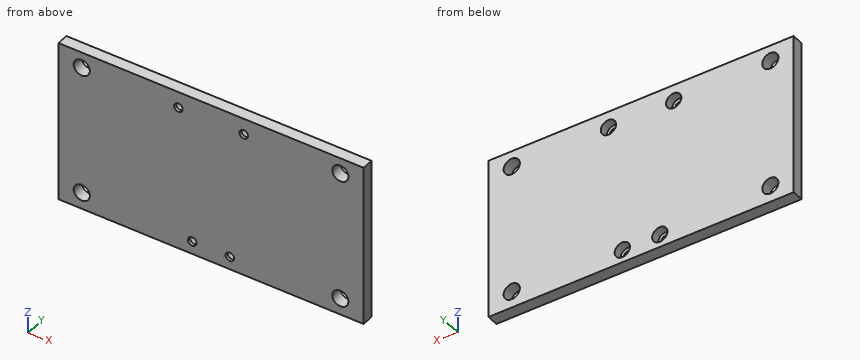
```python
from build123d import *

# Parameters (mm, degrees)
SKETCH1_W                                            = 119.888
SKETCH1_H                                            = 63.5
BOSS_EXTRUDE1_DEPTH                                  = 4.572
CBORE_FOR_M3_HEXAGON_SOCKET_HEAD_CAP_SCR_D           = 3.4
CBORE_FOR_M3_HEXAGON_SOCKET_HEAD_CAP_SCR_CBORE_D     = 6
CBORE_FOR_M3_HEXAGON_SOCKET_HEAD_CAP_SCR_CBORE_DEPTH = 3.4
SKETCH5_R                                            = 3.175
CUT_EXTRUDE1_DEPTH                                   = 5.572


with BuildPart() as part:
    # Sketch1 → Boss-Extrude1 (new body)
    with BuildSketch(Plane(origin=(0, 0, 0), x_dir=(1, 0, 0), z_dir=(0, 1, 0))):
        Rectangle(SKETCH1_W, SKETCH1_H)
    extrude(amount=BOSS_EXTRUDE1_DEPTH)

    # CBORE for M3 Hexagon socket head cap screws1 (through all)
    with Locations(Plane(origin=(0, 4.572, 0), x_dir=(1, 0, 0), z_dir=(0, 1, 0))):
        with Locations((7.366, 26.67), (12.827, -25.4), (-12.827, -25.4), (-7.366, 26.67)):
            CounterBoreHole(CBORE_FOR_M3_HEXAGON_SOCKET_HEAD_CAP_SCR_D / 2, CBORE_FOR_M3_HEXAGON_SOCKET_HEAD_CAP_SCR_CBORE_D / 2, CBORE_FOR_M3_HEXAGON_SOCKET_HEAD_CAP_SCR_CBORE_DEPTH)

    # Sketch5 → Cut-Extrude1 (cut, through all)
    with BuildSketch(Plane(origin=(0, 4.572, 0), x_dir=(1, 0, 0), z_dir=(0, 1, 0))):
        with Locations((50.8, 25.225713352)):
            Circle(SKETCH5_R)
        with Locations((50.8, -25.574286648)):
            Circle(SKETCH5_R)
        with Locations((-50.8, 25.225713352)):
            Circle(SKETCH5_R)
        with Locations((-50.8, -25.574286648)):
            Circle(SKETCH5_R)
    extrude(amount=-CUT_EXTRUDE1_DEPTH, mode=Mode.SUBTRACT)


solid = part.part
```
Work out the finished part from the listing and answer in its coordinate system (mm). Give positions to 0.01 mm unless a question says otherwise; leave off trailing zeros. Loops run counter-clockwise (first coordinate to the right, second up) from the corner with the lowest first, then second, coordinate; pieces in that order, holes last. Notation, with made-up numbers: (-28, 80) - (0, 80) arc R14 cw to (0, 93) - close; hole circle Ø7 at (69.25, 8). An arc over 180 degrees is marked (long way). One line per question, with ' | ' between items.
(1) The part is cut by section B-B (x = -7). Write down the section's boundary in (y, z), then the cut area to 3 significant figures.
Recorded:
outline: (0, -31.75) - (4.57, -31.75) - (4.57, -29.65) - (1.17, -29.65) - (1.17, -28.33) - (0, -28.33) - close; (0, -25.01) - (1.17, -25.01) - (1.17, -23.69) - (4.57, -23.69) - (4.57, 31.75) - (0, 31.75) - close | area: 266 mm²
(2) The part is cut by section C-C (y = 2.25). Count the separate pieces of the cut face and the enclosed holes in it, then the cut area to 3 significant figures.
Recorded:
separate pieces: 1 | enclosed holes: 8 | area: 7,370 mm²
(3) The part is cut by section A-A (x = 50.8). Write down the section's boundary in (y, z).
Recorded:
outline: (0, -31.75) - (4.57, -31.75) - (4.57, -28.4) - (0, -28.4) - close; (0, -22.05) - (4.57, -22.05) - (4.57, 22.4) - (0, 22.4) - close; (0, 28.75) - (4.57, 28.75) - (4.57, 31.75) - (0, 31.75) - close
(4) This flat-tipped pin is pushed along its axis until it touches: pin 1 Ø4.5 at (x, z) = (12.827, 25.4) entering from +Y. Where does it stop, or does it pass through?
Recorded:
pin 1: stops at y = 1.17
(5) Straight lines are drawn through the part: probe 1 along X at (y, z) = (0.6, 25.4); probe 2 along Z at (x, y) = (53, 2.8); probe 3 along X at (y, z) = (3.35, -22.5). For each, find the intervals that lie inside material, in ascending order.
Recorded:
probe 1: x = -59.94 to -53.97, -47.63 to -14.53, -11.13 to 11.13, 14.53 to 47.63, 53.97 to 59.94 | probe 2: z = -31.75 to -27.51, -22.94 to 23.29, 27.86 to 31.75 | probe 3: x = -59.94 to -52.43, -49.17 to 49.17, 52.43 to 59.94
